The listing builds one solid part. Answer for the finished solid, in the listing's coordinates (mm). A direction names the side the tool comes from. Coordinates: 2 decimals unless noted, no trailing zeros. Loops run counter-clockwise (first coordinate to the right, second up) from the corner with the lowest first, then second, coordinate; pieces in that order, holes last. Notation, with made-up numbers: (21, -1.5) - (47, -1.5) arc R38 ccw to (47, 36.5) - close; hole circle Ø11 at (14, 38). An arc over 180 degrees is marked (long way). Return JSON: item names as keys, results as strings. Group by question number.
1. This flat-tipped pin is pushed along its axis until it touches: P1, Ø1.5, axis at x = 7.5, y = 2, coming from the -Z side. Where does it stop, or does it pass through?
2. Find the intervals of material crossed by line 1 along X through (y, z) = (1.55, -1.75); line 2 along Z through (x, y) = (16.5, 0); line 3 along Z through (x, y) = (13.75, 0), in increasing order.
3. Which of the six approach directions +Z, -Z, +X, -X, +Y, -Y give full straight-line access (tool end or side, diameter ignored) to faces 1 (the face through (10, -1, -2)), 2 (the face through (20, -3, 0))?
4. Section A-A (y = 0) is taken. Write down the section's boundary in (x, z), and give its area (3 significant figures).
5. The mould has two halves that part along X. Classify faces 3 (the face through (12, 0, -2)), 4 (the face through (0, -1, 1)), 5 (the face through (5, -3, 0)): pulls with the +X half, pulls with the -X half, needs draft (parallel to the pull), parting line crosses it, or undercut.
6. Section C-C (x = 19.75) is taken. Write down the section's boundary in (y, z), and give its area (3 significant figures).
7. Section D-D (y = -2.3) is taken. Write down the section's boundary in (x, z).
```python
from build123d import *

# Parameters (mm, degrees)
F2_R     = 1
F3_DEPTH = 25.001


with BuildPart() as f1:
    # F0 (on Top) → F1 (revolve)
    with BuildSketch(Plane.XY):
        Polygon((0, 3), (0, 0), (25, 0), (25, 3), (15, 3), (15, 2), (10, 2), (10, 3), align=None)
    revolve(axis=Axis((12.5, 0, 0), (1, 0, 0)))

    # F2 (on face) → F3 (cut, through all)
    with BuildSketch(Plane(origin=(0, 0, 0), x_dir=(0, -1, 0), z_dir=(-1, 0, 0))):
        Circle(F2_R)
    extrude(amount=-F3_DEPTH, mode=Mode.SUBTRACT)


solid = f1.part
```
The answers:
{
 "1": {"P1": "stops at z = -2.73"},
 "2": {"line 1": "x = 0 to 10, 15 to 25", "line 2": "z = -3 to -1, 1 to 3", "line 3": "z = -2 to -1, 1 to 2"},
 "3": {"face 1": "none", "face 2": "+X, -X"},
 "4": {"outline": "(0, -3) - (10, -3) - (10, -2) - (15, -2) - (15, -3) - (25, -3) - (25, -1) - (0, -1) - close; (0, 1) - (25, 1) - (25, 3) - (15, 3) - (15, 2) - (10, 2) - (10, 3) - (0, 3) - close", "area": "90.0 mm2"},
 "5": {"face 3": "undercut", "face 4": "pulls with the -X half", "face 5": "needs draft"},
 "6": {"outline": "circle Ø6 at (0, 0); hole circle Ø2 at (0, 0)", "area": "25.1 mm2"},
 "7": {"outline": "(0, -1.93) - (10, -1.93) - (10, 1.93) - (0, 1.93) - close; (15, -1.93) - (25, -1.93) - (25, 1.93) - (15, 1.93) - close"}
}
